from build123d import *

# Parameters (mm, degrees)
F0_W     = 300
F0_H     = 200
F0_R     = 15
F1_DEPTH = 100
F2_R     = 10


with BuildPart() as f1:
    # F0 (on Top) → F1 (new body)
    with BuildSketch(Plane.XY):
        with Locations((9.53036, 21.334988)):
            Rectangle(F0_W, F0_H)
        with Locations((133.951858, 13.06554)):
            Circle(F0_R, mode=Mode.SUBTRACT)
    extrude(amount=F1_DEPTH)

    # F2
    f2_edges = [f1.edges().sort_by_distance(p)[0] for p in [
        (-140.46964, 121.334988, 50),
    ]]
    fillet(f2_edges, radius=F2_R)


solid = f1.part
Check sheet for the modelled part. Datum: model origin and axes. Units: mm. Round coordinates to 2 decimals unless told otherwise and drop trailing zeros. Loops run counter-clockwise (first coordinate to the right, second up) from the corner with the lowest first, then second, coordinate; pieces in that order, holes last. Notation, with made-up numbers: (59.25, 10) -> (76.25, 10) arc R32 ccw to (76.25, 37) -> close; hole circle Ø7 at (43, 56). An arc over 180 degrees is marked (long way). Put each result on its own line as item: value. Start each with the question number.
1. Scan lines: probe 1 along Y at (x, z) = (135, 37); probe 2 along X at (y, z) = (4, 80.5); probe 3 along X at (y, z) = (17, 91). Record each from-to range of solid material in increasing order.
2. Section check A-A (y = 8.5). Enter the section's corners in (x, z), plus the area to 3 significant figures.
3. Gauge pin test, flat end, axial feed: pin 1 (24 mm diameter, centred on x = 133.95, y = 13.07, fed in from -Z). Record the tip position at first contact, or that the pin passes through.
4. Draft check along Y on faces 1 (the face through (148.26, 17.57, 49.3)), 2 (the face through (7, -78.665, 49)), 3 (the face through (-140.47, 15, 49)), 4 (the face through (-137.618, 118.328, 50.7)). Enter one of: +Y half, -Y half, draft (parallel to the pull), parting line (faces both ways), or undercut.
Findings:
1. probe 1: y = -78.67 to -1.9, 28.03 to 121.33
1. probe 2: x = -140.47 to 122, 145.9 to 159.53
1. probe 3: x = -140.47 to 119.48, 148.43 to 159.53
2. outline: (-140.47, 0) -> (119.66, 0) -> (119.66, 100) -> (-140.47, 100) -> close; (148.24, 0) -> (159.53, 0) -> (159.53, 100) -> (148.24, 100) -> close
2. area: 27,100 mm^2
3. pin 1: passes through
4. face 1: undercut
4. face 2: -Y half
4. face 3: draft
4. face 4: +Y half
